The listing builds one solid part. Answer for the finished solid, in the listing's coordinates (mm). A direction names the side the tool comes from. Give positions to 0.01 mm unless a question says otherwise; leave off trailing zeros. Loops run counter-clockwise (first coordinate to the right, second up) from the corner with the lowest first, then second, coordinate; pieces in that order, holes last.
Item 1: The mould has two halves that part along X. Classify faces 5 (the face through (-13.92, 3, 4)), 6 (the face through (-15.25, -18, 1)), 7 (the face through (0, 27.41, 1)), 8 (the face through (17.931, -14.542, 1.252)): pulls with the +X half, pulls with the -X half, needs draft (parallel to the pull), parting line crosses it, or undercut.
Item 2: Section C-C, the plane y = 4.5 is taken. Give the vertices of the cut face in (x, z).
Item 3: Consider line 1 along X through (y, z) = (4, 4.25); line 2 along X through (y, z) = (-11.5, 1.5); line 3 along Y through (x, z) = (15, 0.75). Determine where each line is inside the solid, lowest interval first.
Item 4: Section B-B, the plane x = 8 is taken. Give the vertices of the cut face in (y, z), and give its area (3 significant figures).
Item 5: A tool of negligible diameter and unlimited length cuts with its end or side. For faces 1 (the face through (-16, 12.335, 4)), 2 (the face through (-13.379, 4, 4)), 3 (the face through (-16, 3, 5.08)), 4 (the face through (-15.25, 25, 1)), from which of +Z, -Z, +X, -X, +Y, -Y can it reach the whole face along a straight path? Write none if from no direction.
Item 6: Each of these flat-tipped pins is pushed along its axis until it touches: pin 1 Ø0.8 at (y, z) = (23.5, 1.5) entering from +X; pin 2 Ø0.8 at (x, z) = (-17.5, 3.5) entering from -Y; pin 3 Ø4 at (x, y) = (13, 22) entering from +Z. Where does it stop, or does it pass through?
Item 7: Section A-A, the plane z = 1.75 is taken. Give the vertices of the cut face in (x, y).
Item 8: Section D-D, the plane y = -15 is taken. Give the vertices of the cut face in (x, z), and give its area (3 significant figures).
Autodesk Inventor part; units mm, degrees
ref_plane "YZ Plane" through (0, 0, 0) normal (1, 0, 0) x (0, 1, 0)
ref_plane "XZ Plane" through (0, 0, 0) normal (0, 1, 0) x (-1, 0, 0)
ref_plane "XY Plane" through (0, 0, 0) normal (0, 0, 1) x (1, 0, 0)
sketch "Sketch1" plane through (0, 0, 0) normal (0, 0, 1) x (1, 0, 0)
  arc A0 (15.6734, 13.8392) -> (14.75, 12.1537) centre (16.75, 12.1537) ccw construction
  line L0 (15.6734, 13.8392) -> (18.0766, 15.3743) construction
  arc A1 (18.0766, 15.3743) -> (19, 17.0598) centre (17, 17.0598) ccw construction
  line L1 (19, 17.0598) -> (19, 30.7058) construction
  arc A2 (24.5861, 42.384) -> (19, 30.7058) centre (34, 30.7058) ccw construction
  line L2 (24.5861, 42.384) -> (28.2876, 45.3677) construction
  arc A3 (28.2876, 45.3677) -> (28.7404, 49.5861) centre (26.4048, 47.7034) ccw construction
  line L3 (28.7404, 49.5861) -> (26.2301, 52.7003) construction
  arc A4 (26.2301, 52.7003) -> (22.0117, 53.1532) centre (23.8944, 50.8175) ccw construction
  line L4 (22.0117, 53.1532) -> (11.4653, 44.6517) construction
  arc A5 (2.0515, 41.3299) -> (11.4653, 44.6517) centre (2.0515, 56.3299) ccw construction
  line L5 (2.0515, 41.3299) -> (-2.0515, 41.3299) construction
  arc A6 (-11.4653, 44.6517) -> (-2.0515, 41.3299) centre (-2.0515, 56.3299) ccw construction
  line L6 (-11.4653, 44.6517) -> (-22.0117, 53.1532) construction
  arc A7 (-22.0117, 53.1532) -> (-26.2301, 52.7003) centre (-23.8944, 50.8175) ccw construction
  line L7 (-26.2301, 52.7003) -> (-28.7404, 49.5861) construction
  arc A8 (-28.7404, 49.5861) -> (-28.2876, 45.3677) centre (-26.4048, 47.7034) ccw construction
  line L8 (-28.2876, 45.3677) -> (-24.5861, 42.384) construction
  arc A9 (-19, 30.7058) -> (-24.5861, 42.384) centre (-34, 30.7058) ccw construction
  line L9 (-19, 30.7058) -> (-19, 17.0598) construction
  arc A10 (-19, 17.0598) -> (-18.0766, 15.3743) centre (-17, 17.0598) ccw construction
  line L10 (-18.0766, 15.3743) -> (-15.6734, 13.8392) construction
  arc A11 (-14.75, 12.1537) -> (-15.6734, 13.8392) centre (-16.75, 12.1537) ccw construction
  line L11 (-14.75, 12.1537) -> (-14.75, -5.494) construction
  arc A12 (-15.6734, -7.1795) -> (-14.75, -5.494) centre (-16.75, -5.494) ccw construction
  line L12 (-15.6734, -7.1795) -> (-18.0766, -8.7146) construction
  arc A13 (-18.0766, -8.7146) -> (-19, -10.4001) centre (-17, -10.4001) ccw construction
  line L13 (-19, -10.4001) -> (-19, -30.7058) construction
  arc A14 (-24.5861, -42.384) -> (-19, -30.7058) centre (-34, -30.7058) ccw construction
  line L14 (-24.5861, -42.384) -> (-28.2876, -45.3677) construction
  arc A15 (-28.2876, -45.3677) -> (-28.7404, -49.5861) centre (-26.4048, -47.7034) ccw construction
  line L15 (-28.7404, -49.5861) -> (-26.2301, -52.7003) construction
  arc A16 (-26.2301, -52.7003) -> (-22.0117, -53.1532) centre (-23.8944, -50.8175) ccw construction
  line L16 (-22.0117, -53.1532) -> (-11.4653, -44.6517) construction
  arc A17 (-2.0515, -41.3299) -> (-11.4653, -44.6517) centre (-2.0515, -56.3299) ccw construction
  line L17 (-2.0515, -41.3299) -> (2.0515, -41.3299) construction
  arc A18 (11.4653, -44.6517) -> (2.0515, -41.3299) centre (2.0515, -56.3299) ccw construction
  line L18 (11.4653, -44.6517) -> (22.0117, -53.1532) construction
  arc A19 (22.0117, -53.1532) -> (26.2301, -52.7003) centre (23.8944, -50.8175) ccw construction
  line L19 (26.2301, -52.7003) -> (28.7404, -49.5861) construction
  arc A20 (28.7404, -49.5861) -> (28.2876, -45.3677) centre (26.4048, -47.7034) ccw construction
  line L20 (28.2876, -45.3677) -> (24.5861, -42.384) construction
  arc A21 (19, -30.7058) -> (24.5861, -42.384) centre (34, -30.7058) ccw construction
  line L21 (19, -30.7058) -> (19, -10.4001) construction
  arc A22 (19, -10.4001) -> (18.0766, -8.7146) centre (17, -10.4001) ccw construction
  line L22 (18.0766, -8.7146) -> (15.6734, -7.1795) construction
  arc A23 (14.75, -5.494) -> (15.6734, -7.1795) centre (16.75, -5.494) ccw construction
  line L23 (14.75, -5.494) -> (14.75, 12.1537) construction
  spline S0 degree 3 poles (8.2673, 8.7575) (8.2937, 7.6146) (8.3178, 6.4713) (8.3615, 4.1764) (8.3811, 3.024) (8.3985, 1.872) knots 0 0 0 0 0.342955 0.342955 0.688597 0.688597 0.688597 0.688597 construction
  arc A24 (7.2587, 0.991) -> (8.3985, 1.872) centre (7.4986, 1.8584) ccw construction
  line L24 (7.2587, 0.991) -> (3.6122, 1.9996) construction
  arc A25 (3.0306, 3.4932) -> (3.6122, 1.9996) centre (3.8788, 2.9634) ccw construction
  line L25 (3.0306, 3.4932) -> (6.6042, 9.2136) construction
  arc A26 (8.2673, 8.7575) -> (6.6042, 9.2136) centre (7.3675, 8.7367) ccw construction
  line L26 (-3.336, -2.3124) -> (-0.2664, -1.464) construction
  arc A27 (0.2664, -1.464) -> (-0.2664, -1.464) centre (0, -2.4278) ccw construction
  line L27 (0.2664, -1.464) -> (3.336, -2.3124) construction
  arc A28 (3.9177, -3.8061) -> (3.336, -2.3124) centre (3.0696, -3.2763) ccw construction
  line L28 (3.9177, -3.8061) -> (0.8481, -8.7198) construction
  arc A29 (-0.8481, -8.7198) -> (0.8481, -8.7198) centre (0, -8.19) ccw construction
  line L29 (-0.8481, -8.7198) -> (-3.9177, -3.8061) construction
  arc A30 (-3.336, -2.3124) -> (-3.9177, -3.8061) centre (-3.0696, -3.2763) ccw construction
  line L30 (6.2794, 18.6976) -> (1.9507, 19.9359) construction
  arc A31 (1.3777, 21.4271) -> (1.9507, 19.9359) centre (2.2258, 20.8973) ccw construction
  line L31 (1.3777, 21.4271) -> (4.6803, 26.7137) construction
  arc A32 (6.5163, 26.3393) -> (4.6803, 26.7137) centre (5.5284, 26.1839) ccw construction
  line L32 (6.5163, 26.3393) -> (7.5423, 19.8143) construction
  arc A33 (6.2794, 18.6976) -> (7.5423, 19.8143) centre (6.5544, 19.659) ccw construction
  line L33 (0.275, 16.6432) -> (4.3044, 15.4905) construction
  arc A34 (4.8775, 13.9992) -> (4.3044, 15.4905) centre (4.0294, 14.529) ccw construction
  line L34 (4.8775, 13.9992) -> (0.8481, 7.5492) construction
  arc A35 (-0.8481, 7.5492) -> (0.8481, 7.5492) centre (0, 8.0791) ccw construction
  line L35 (-0.8481, 7.5492) -> (-4.8775, 13.9992) construction
  arc A36 (-4.3044, 15.4905) -> (-4.8775, 13.9992) centre (-4.0294, 14.529) ccw construction
  line L36 (-4.3044, 15.4905) -> (-0.275, 16.6432) construction
  arc A37 (0.275, 16.6432) -> (-0.275, 16.6432) centre (0, 15.6817) ccw construction
  spline S1 degree 3 poles (-8.3985, 1.872) (-8.3811, 3.024) (-8.3615, 4.1764) (-8.3178, 6.4713) (-8.2937, 7.6146) (-8.2673, 8.7575) knots 0 0 0 0 0.345643 0.345643 0.688601 0.688601 0.688601 0.688601 construction
  arc A38 (-6.6042, 9.2136) -> (-8.2673, 8.7575) centre (-7.3675, 8.7367) ccw construction
  line L37 (-6.6042, 9.2136) -> (-3.0306, 3.4932) construction
  arc A39 (-3.6122, 1.9996) -> (-3.0306, 3.4932) centre (-3.8788, 2.9634) ccw construction
  line L38 (-3.6122, 1.9996) -> (-7.2587, 0.991) construction
  arc A40 (-8.3985, 1.872) -> (-7.2587, 0.991) centre (-7.4986, 1.8584) ccw construction
  line L39 (-4.6803, 26.7137) -> (-1.3777, 21.4271) construction
  arc A41 (-1.9507, 19.9359) -> (-1.3777, 21.4271) centre (-2.2258, 20.8973) ccw construction
  line L40 (-1.9507, 19.9359) -> (-6.2794, 18.6976) construction
  arc A42 (-7.5423, 19.8143) -> (-6.2794, 18.6976) centre (-6.5544, 19.659) ccw construction
  line L41 (-7.5423, 19.8143) -> (-6.5163, 26.3393) construction
  arc A43 (-4.6803, 26.7137) -> (-6.5163, 26.3393) centre (-5.5284, 26.1839) ccw construction
  circle A44 centre (-23.5925, -48.0053) radius 1.475 construction
  arc A45 (3, -16.1701) -> (-3, -16.1701) centre (0, -16.1701) ccw construction
  line L42 (3, -16.1701) -> (3, -28.3299) construction
  arc A46 (-3, -28.3299) -> (3, -28.3299) centre (0, -28.3299) ccw construction
  line L43 (-3, -28.3299) -> (-3, -16.1701) construction
  circle A47 centre (-23.5925, 48.0053) radius 1.475 construction
  circle A48 centre (-10, 13.3299) radius 1.475 construction
  circle A49 centre (-10, -6.6701) radius 1.475 construction
  circle A50 centre (-15.25, -11.9201) radius 1.5
  circle A51 centre (-14.25, -40.4742) radius 1.475 construction
  circle A52 centre (23.5925, -48.0053) radius 1.475 construction
  circle A53 centre (15.25, -11.9201) radius 1.5
  circle A54 centre (14.25, 40.4742) radius 1.475 construction
  circle A55 centre (10, 13.3299) radius 1.475 construction
  circle A56 centre (14.25, -40.4742) radius 1.475 construction
  circle A57 centre (15.25, 18.5799) radius 1.5
  circle A58 centre (-15.25, 18.5799) radius 1.5
  circle A59 centre (10, -6.6701) radius 1.475 construction
  circle A60 centre (-14.25, 40.4742) radius 1.475 construction
  circle A61 centre (23.5925, 48.0053) radius 1.475 construction
  line L44 (19, 22.3299) -> (15.25, 22.3299) construction
  line L45 (-19, 22.3299) -> (-19, 18.5799) construction
  line L46 (-19, -15.6701) -> (-15.25, -15.6701) construction
  line L47 (19, -15.6701) -> (19, -11.9201) construction
  arc A62 (19, 18.5799) -> (15.25, 22.3299) centre (15.25, 18.5799) ccw
  arc A63 (-15.25, 22.3299) -> (-19, 18.5799) centre (-15.25, 18.5799) ccw
  arc A64 (15.25, -15.6701) -> (19, -11.9201) centre (15.25, -11.9201) ccw
  arc A65 (-19, -11.9201) -> (-15.25, -15.6701) centre (-15.25, -11.9201) ccw
  arc A66 (-19, 18.5799) -> (-15.25, 22.3299) centre (-15.25, 18.5799) ccw construction
  arc A67 (15.25, 22.3299) -> (19, 18.5799) centre (15.25, 18.5799) ccw construction
  arc A68 (19, -11.9201) -> (15.25, -15.6701) centre (15.25, -11.9201) ccw construction
  arc A69 (-15.25, -15.6701) -> (-19, -11.9201) centre (-15.25, -11.9201) ccw construction
  line L48 (19, 18.5799) -> (19, 22.3299) construction
  line L49 (15.25, 22.3299) -> (-15.25, 22.3299)
  line L50 (-15.25, 22.3299) -> (-19, 22.3299) construction
  line L51 (-19, 18.5799) -> (-19, -11.9201)
  line L52 (-19, -11.9201) -> (-19, -15.6701) construction
  line L53 (-15.25, -15.6701) -> (15.25, -15.6701)
  line L54 (15.25, -15.6701) -> (19, -15.6701) construction
  line L55 (19, -11.9201) -> (19, 18.5799)
  point P0 (0, 0)
  dimension "d0" = 3.75
  dimension "d1" = 3.75
  dimension "d2" = 3.75
extrude "Extrusion1" add sketch "Sketch1" along normal blind 2.54
sketch "Sketch2" plane through (0, 0, 2.54) normal (0, 0, 1) x (1, 0, 0)
  line L0 (-13.92, 12.3346) -> (-19, 12.3346)
  line L1 (-19, 12.3346) -> (-19, -5.6749)
  line L2 (-19, -5.6749) -> (-13.92, -5.6749)
  line L3 (-13.92, -5.6749) -> (-13.92, 12.3346)
  line L4 (15.25, 22.3299) -> (-15.25, 22.3299) construction
  line L5 (-15.25, -15.6701) -> (15.25, -15.6701) construction
  line L6 (-19, 18.5799) -> (-19, -11.9201) construction
  point P0 (0, 0)
  dimension "d5" = 9.9953
  dimension "d6" = 9.9953
  dimension "d7" = 5.08
extrude "Extrusion2" add sketch "Sketch2" along normal blind 2.54
sketch "Sketch3" plane through (0, 0, 2.54) normal (0, 0, 1) x (1, 0, 0)
  line L0 (19, -11.9201) -> (19, 18.5799)
  line L1 (19, 15.9799) -> (-13.3786, 15.9799)
  line L2 (-13.3786, 15.9799) -> (-13.3786, -9.3201)
  line L3 (-13.3786, -9.3201) -> (19, -9.3201)
  line L4 (19, -9.3201) -> (19, 15.9799)
  line L5 (15.25, 22.3299) -> (-15.25, 22.3299)
  line L6 (-15.25, -15.6701) -> (15.25, -15.6701)
  point P0 (0, 0)
  dimension "d10" = 6.35
  dimension "d11" = 6.35
extrude "Extrusion3" add sketch "Sketch3" along normal blind 3.556
chamfer "Chamfer1" distance 3.175 angle 45 1 edges at (2.8107, 15.9799, 6.096)
chamfer "Chamfer2" distance 3.175 angle 45 1 edges at (2.8107, -9.3201, 6.096)
sketch "Sketch4" plane through (-15.25, 22.3299, 0) normal (0, 1, 0) x (1, 0, 0)
  line L0 (30.5, 0) -> (0, 0)
  line L1 (0, 0) -> (0, -2.54)
  line L2 (30.5, -2.54) -> (0, -2.54)
  line L3 (30.5, 0) -> (30.5, -2.54)
  point P0 (15.25, 0)
extrude "Extrusion4" add sketch "Sketch4" along normal blind 5.08
sketch "Sketch5" plane through (-15.25, -15.6701, 0) normal (0, -1, 0) x (1, 0, 0)
  line L0 (0, 0) -> (30.5, 0)
  line L1 (30.5, 0) -> (30.5, 2.54)
  line L2 (0, 2.54) -> (30.5, 2.54)
  line L3 (0, 0) -> (0, 2.54)
  point P0 (15.25, 0)
extrude "Extrusion5" add sketch "Sketch5" along normal blind 5.08
equation "\"d1\" = d0"
equation "\"d2\" = d0"
equation "\"d6\" = d5"
equation "\"d11\" = d10"
properties part number "Velox ESC"
Worked answers:
1. face 5: undercut
1. face 6: pulls with the -X half
1. face 7: needs draft
1. face 8: pulls with the +X half
2. outline: (-19, 0) - (19, 0) - (19, 6.1) - (-13.38, 6.1) - (-13.38, 2.54) - (-13.92, 2.54) - (-13.92, 5.08) - (-19, 5.08) - close
3. line 1: x = -19 to -13.92, -13.38 to 19
3. line 2: x = -19 to -16.69, -13.81 to 13.81, 16.69 to 19
3. line 3: y = -20.75 to -13.4, -10.44 to 17.1, 20.06 to 27.41
4. outline: (-20.75, 0) - (27.41, 0) - (27.41, 2.54) - (15.98, 2.54) - (15.98, 2.92) - (12.8, 6.1) - (-6.15, 6.1) - (-9.32, 2.92) - (-9.32, 2.54) - (-20.75, 2.54) - close
4. area: 202 mm2
5. face 1: +Z, -X, +Y
5. face 2: +Z, +Y, -Y
5. face 3: +Z, -X, +Y, -Y
5. face 4: +Z, -Z, -X, +Y
6. pin 1: stops at x = 15.25
6. pin 2: stops at y = -5.67
6. pin 3: stops at z = 2.54
7. outline: (-19, -11.92) arc R3.75 ccw to (-15.25, -15.67) - (-15.25, -20.75) - (15.25, -20.75) - (15.25, -15.67) arc R3.75 ccw to (19, -11.92) - (19, 18.58) arc R3.75 ccw to (15.25, 22.33) - (15.25, 27.41) - (-15.25, 27.41) - (-15.25, 22.33) arc R3.75 ccw to (-19, 18.58) - close; hole circle Ø3 at (-15.25, -11.92); hole circle Ø3 at (-15.25, 18.58); hole circle Ø3 at (15.25, -11.92); hole circle Ø3 at (15.25, 18.58)
8. outline: (-17.39, 0) - (17.39, 0) - (17.39, 2.54) - (-17.39, 2.54) - close
8. area: 88.3 mm2
